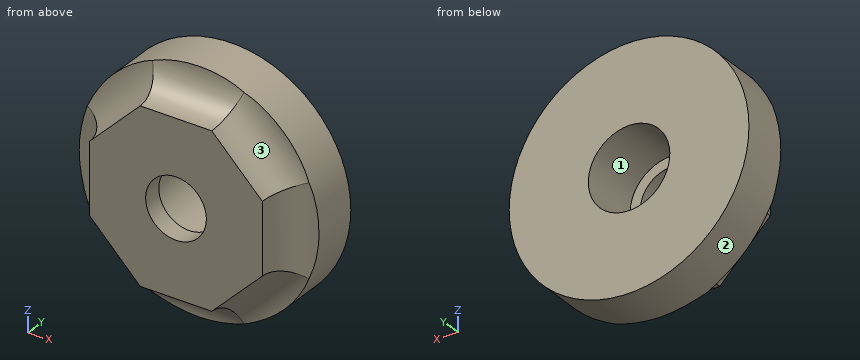
Autodesk Inventor part; units mm, degrees
ref_plane "YZ Plane" through (0, 0, 0) normal (1, 0, 0) x (0, 1, 0)
ref_plane "XZ Plane" through (0, 0, 0) normal (0, 1, 0) x (-1, 0, 0)
ref_plane "XY Plane" through (0, 0, 0) normal (0, 0, 1) x (1, 0, 0)
sketch "Sketch1" plane through (0, 0, 0) normal (0, 1, 0) x (-1, 0, 0)
  circle A0 centre (0, 0) radius 7.5
  dimension "d0" = 15
extrude "Extrusion1" add sketch "Sketch1" along normal blind 5
sketch "Sketch2" plane through (0, 0, 0) normal (0, 0, 1) x (1, 0, 0)
  line L0 (-7.5, 0) -> (7.5, 0)
  line L1 (0, 0) -> (7.5, 0)
  circle A0 centre (7.5, 0) radius 2.1
  dimension "d3" = 4.2
extrude "Extrusion2" cut sketch "Sketch2" along normal mid plane 8
pattern_circular "Circular Pattern1" count 8 over 360 about axis through (0, 0, 0) along (0, 1, 0) of "Extrusion2"
sketch "Sketch3" plane through (0, 5, 0) normal (0, 1, 0) x (1, 0, 0)
  circle A0 centre (0, 0) radius 2.55
  dimension "d9" = 5.1
hole "Hole1" at (0, 5, 0) direction (0, -1, 0) diameter 3.8 end through all counterbore diameter 5.1 counterbore depth 3.8
properties part number "Restraining_cylinder"
Read the model definition and answer for the solid it produces. Units are mm, in the model's axes. Face numbers are marked on the shaded views. Coordinates: 2 decimals unless noted, no trailing zeros. Write each loop counter-clockwise with the first axis right and the second up, starting at its lowest first coordinate (ties: lowest second). Pieces come first, ordered by that corner, then holes. Notation, with made-up numbers: (-36.75, 32.5) -> (20.25, 32.5) arc R6 ccw to (20.25, 38.5) -> close; hole circle Ø9 at (-20, 4.25). An arc over 180 degrees is marked (long way). Return JSON: item names as keys, results as strings.
1. Each of these flat-tipped pins is pushed along its axis until it touches: P1, Ø5, axis at x = 0, z = 0, coming from the +Y side; P2, Ø3, axis at x = 0, z = 0, coming from the -Y side. Where does it stop, or does it pass through?
Found:
{"P1": "y = 1.2", "P2": "through"}
2. A cutting plane is placed at A-A (z = 0). Determine the outline of the cut face in (x, y), and give its area (3 significant figures).
Found:
{"outline": "(-7.5, 2.1) arc R2.1 cw to (-5.4, 0) -> (-1.9, 0) -> (-1.9, 1.2) -> (-2.55, 1.2) -> (-2.55, 5) -> (-7.5, 5) -> close; (1.9, 0) -> (5.4, 0) arc R2.1 cw to (7.5, 2.1) -> (7.5, 5) -> (2.55, 5) -> (2.55, 1.2) -> (1.9, 1.2) -> close", "area": "44.1 mm2"}
3. A cutting plane is placed at C-C (y = 2.5). Determine the outline of the cut face in (x, z), and give its area (3 significant figures).
Found:
{"outline": "circle Ø15 at (0, 0); hole circle Ø5.1 at (0, 0)", "area": "156 mm2"}
4. Determine the mould class of the marked faces 1, 2 and 3 for opening direction X: pulls with the +X half, pulls with the -X half, needs draft (parallel to the pull), parting line crosses it, or undercut.
Found:
{"face 1": "undercut", "face 2": "parting line crosses it", "face 3": "pulls with the +X half"}
5. A cutting plane is placed at B-B (x = 0). Determine the outline of the cut face in (y, z), and give its area (3 significant figures).
Found:
{"outline": "(0, -5.4) arc R2.1 cw to (2.1, -7.5) -> (5, -7.5) -> (5, -2.55) -> (1.2, -2.55) -> (1.2, -1.9) -> (0, -1.9) -> close; (0, 1.9) -> (1.2, 1.9) -> (1.2, 2.55) -> (5, 2.55) -> (5, 7.5) -> (2.1, 7.5) arc R2.1 cw to (0, 5.4) -> close", "area": "44.1 mm2"}
6. Find the intervals of material crossed by line 1 along X through (y, z) = (3, 0); line 2 along X through (y, z) = (4.15, -2.25), in increasing order. Write a range as from..to.
Found:
{"line 1": "-7.5..-2.55, 2.55..7.5", "line 2": "-7.15..-1.2, 1.2..7.15"}
